Verification items for the finished model (mm, model axes). A direction names the side the tool comes from. Coordinates: 2 decimals unless noted, no trailing zeros. Order: outer loops, then holes, each group sorted by start corner. A loop starts at its lowest first (then second) coordinate and runs counter-clockwise, first axis right, second up.
Q1. Cross-section at C-C, the plane y = -0.5. Record the boundary of the cut face in (x, z), and give its area (3 significant figures).
Q2. Depth check by flat-ended pin: P1, Ø1.9, axis at x = -1.5, y = 1.5, coming from the +Z side; P2, Ø1.6, axis at x = 2.5, z = 7, coming from the +Y side; P3, Ø1.6, axis at x = 0.5, z = 4, coming from the +Y side. Enter the tip coordinate at first touch or a pass-through.
Q3. Cross-section at A-A, the plane x = 0. Record the boundary of the cut face in (y, z), and give its area (3 significant figures).
Q4. Set-up check for faces 1 (the flat face through (-0.1, 2.4, 6)), 2 (the flat face through (4, 4, 1)), 3 (the flat face through (1, 3.4, 4.5)), 4 (the cylindrical face through (0, -4, 5)), 5 (the flat face through (-2.2, 0.1, 0)): record each of +Z, -Z, +X, -X, +Y, -Y from which the full face is reachable in a straight line by a thin tool's end or side.
Q5. Draft check along Y on faces 6 (the flat face through (0.1, 3.4, 3)), 7 (the flat face through (-4, 4, 1)), 8 (the cylindrical face through (0, -2, 3)). Enter one of: pulls with the +Y half, pulls with the -Y half, needs draft (parallel to the pull), parting line crosses it, or undercut.
Q6. Thickness scan on line 1 (Y direction, x = 0, z = 4.25); line 2 (Y direction, x = 0, z = 1); line 3 (Z direction, x = 0.75, y = 3.75). Record the ranges inside material, lowest first.
Q7. Cross-section at D-D, the plane y = -3.25. Record the boundary of the cut face in (x, z).
Q8. Cross-section at B-B, the plane z = 2. Record the boundary of the cut face in (x, y), and give its area (3 significant figures).
from build123d import *

# Parameters (mm, degrees)
SKETCH2_R           = 2
BOSS_EXTRUDE1_DEPTH = 3
SKETCH3_R           = 2
BOSS_EXTRUDE2_DEPTH = 6
SKETCH4_W           = 8
SKETCH4_H           = 4.603389885
CUT_EXTRUDE1_DEPTH  = 3


with BuildPart() as part:
    # Sketch2 → Boss-Extrude1 (new body)
    with BuildSketch(Plane.XY):
        Polygon((-5, 3), (-3, 5), (3, 5), (5, 3), (5, -3), (3, -5), (-3, -5), (-5, -3), align=None)
        Circle(SKETCH2_R, mode=Mode.SUBTRACT)
    extrude(amount=BOSS_EXTRUDE1_DEPTH)

    # Sketch3 → Boss-Extrude2 (add)
    with BuildSketch(Plane.XY.offset(3)):
        with BuildLine():
            Line((1, 3), (-1, 3))
            Line((-1, 3), (-1, 3.872983346))
            ThreePointArc((-1, 3.872983346), (0, -4), (1, 3.872983346))
            Line((1, 3.872983346), (1, 3))
        make_face()
        Circle(SKETCH3_R, mode=Mode.SUBTRACT)
    extrude(amount=BOSS_EXTRUDE2_DEPTH)

    # Sketch4 → Cut-Extrude1 (cut)
    with BuildSketch(Plane.XY.offset(9)):
        with Locations((0, 2.301694943)):
            Rectangle(SKETCH4_W, SKETCH4_H)
    extrude(amount=-CUT_EXTRUDE1_DEPTH, mode=Mode.SUBTRACT)


solid = part.part
Check values:
1. outline: (-5, 0) - (-1.94, 0) - (-1.94, 9) - (-3.97, 9) - (-3.97, 3) - (-5, 3) - close; (1.94, 0) - (5, 0) - (5, 3) - (3.97, 3) - (3.97, 9) - (1.94, 9) - close
1. area: 42.8 mm2
2. P1: stops at z = 6
2. P2: stops at y = 0
2. P3: stops at y = 3.87
3. outline: (-5, 0) - (-2, 0) - (-2, 9) - (-4, 9) - (-4, 3) - (-5, 3) - close; (2, 0) - (5, 0) - (5, 3) - (3, 3) - (3, 6) - (2, 6) - close
3. area: 33.0 mm2
4. face 1: +Z, +X, -X, +Y
4. face 2: +Z, -Z, +X, +Y
4. face 3: +Z, +Y
4. face 4: +Z
4. face 5: -Z, +X, -X, +Y, -Y
5. face 6: needs draft
5. face 7: pulls with the +Y half
5. face 8: undercut
6. line 1: y = -4 to -2, 2 to 3
6. line 2: y = -5 to -2, 2 to 5
6. line 3: z = 0 to 3
7. outline: (-4.75, 0) - (4.75, 0) - (4.75, 3) - (2.33, 3) - (2.33, 9) - (-2.33, 9) - (-2.33, 3) - (-4.75, 3) - close
8. outline: (-5, -3) - (-3, -5) - (3, -5) - (5, -3) - (5, 3) - (3, 5) - (-3, 5) - (-5, 3) - close; hole circle Ø4 at (0, 0)
8. area: 79.4 mm2
